Read the model definition and answer for the solid it produces. Units are mm, in the model's axes. A direction names the side the tool comes from. Give positions to 0.01 mm unless a question says otherwise; leave off trailing zeros. Order: outer loops, then holes, each group sorted by start corner. A loop starts at its lowest first (then second) coordinate and runs counter-clockwise, first axis right, second up. Notation, with made-up numbers: (72, -3.75) - (126, -3.75) arc R22 cw to (126, 10.25) - close; hole circle Ø10 at (70, 44.25). An arc over 180 degrees is marked (long way). Use a Markdown table: item, result. Add a question column.
1. For a pull along Y with two mould halves and no side action, classify faces 3 (the cylindrical face through (41, 3, 0)), 4 (the flat face through (29, 6, -15.218)), 5 (the flat face through (29, 8.5, -62)), 6 (the cylindrical face through (28.594, -0.003, -0.539)) as released by +Y, released by -Y, zero draft, split by the parting line, or undercut.
2. A cutting plane is placed at D-D on x = 25.5. Determine the outline of the cut face in (y, z).
3. A cutting plane is placed at C-C on y = -1.75. Determine the outline of the cut face in (x, z), and give its area (3 significant figures).
4. Which of the six approach directions +Z, -Z, +X, -X, +Y, -Y give full straight-line access (tool end or side, diameter ignored) to faces 1 (the cylindrical face through (28.59, -2.46, -27.39)), 2 (the flat face through (29, -13, -36))?
5. Flat-ended cylindrical pins translate along their axes: P1, Ø1.7, axis at x = 41, y = 5.5, coming from the -Z side; P2, Ø2.5, axis at x = 15, z = 0, coming from the +Y side; P3, Ø1, axis at x = 6, z = -7, coming from the -Y side; P4, Ø10, axis at x = 21, z = -8.5, coming from the -Y side. Find the tip coordinate at first contact, or state that the pin passes through.
6. Consider L1, parallel to X at y = 2.9, z = 0; L2, parallel to Y at x = 26.5, z = -69; L3, parallel to Z at x = 44, y = 11.5. Determine where each line is inside the solid, lowest interval first.
7. A cutting plane is placed at B-B on x = 43. Determine the outline of the cut face in (y, z), and give its area (3 significant figures).
8. A cutting plane is placed at A-A on z = 0. Determine the outline of the cut face in (x, y).
```python
from build123d import *

# Parameters (mm, degrees)
BOSS_EXTRUDE2_DEPTH     = 58
SKETCH4_R               = 2
CUT_EXTRUDE2_DEPTH      = 58
CUT_EXTRUDE2_DEPTH_BACK = 58


with BuildPart() as part:
    # Sketch3 → Boss-Extrude2 (new body)
    with BuildSketch(Plane(origin=(0, 0, 0), x_dir=(0, 0, -1), z_dir=(1, 0, 0))):
        with BuildLine():
            Line((-34.648232278, -14.351767722), (-38.183766184, -10.816233816))
            ThreePointArc((-38.183766184, -10.816233816), (-15.829835797, 2.627669894), (10.217922448, 4.024466625))
            Line((10.217922448, 4.024466625), (10.217922448, 13.5))
            Line((10.217922448, 13.5), (108, 13.5))
            Line((108, 13.5), (108, 8.5))
            Line((108, 8.5), (15.217922448, 8.5))
            Line((15.217922448, 8.5), (15.217922448, 2.811338878))
            ThreePointArc((15.217922448, 2.811338878), (27.556537728, -2.560391599), (38.183766184, -10.816233816))
            Line((38.183766184, -10.816233816), (34.648232278, -14.351767722))
            ThreePointArc((34.648232278, -14.351767722), (0, 0), (-34.648232278, -14.351767722))
        make_face()
    extrude(amount=BOSS_EXTRUDE2_DEPTH)

    # Sketch4 → Cut-Extrude2 (cut, two sides)
    with BuildSketch(Plane(origin=(0, 0, 0), x_dir=(1, 0, 0), z_dir=(0, 1, 0))) as cut_extrude2_sk:
        with Locations((15, 0)):
            Circle(SKETCH4_R)
        with Locations((43, 0)):
            Circle(SKETCH4_R)
    extrude(amount=CUT_EXTRUDE2_DEPTH, mode=Mode.SUBTRACT)
    extrude(cut_extrude2_sk.sketch, amount=-CUT_EXTRUDE2_DEPTH_BACK, mode=Mode.SUBTRACT)


solid = part.part
```
Output values:
| question | item | result |
|---|---|---|
| 1 | face 3 | zero draft |
| 1 | face 4 | undercut |
| 1 | face 5 | undercut |
| 1 | face 6 | released by -Y |
| 2 | outline | (-14.35, -34.65) - (-10.82, -38.18) arc R54 ccw to (2.81, -15.22) - (8.5, -15.22) - (8.5, -108) - (13.5, -108) - (13.5, -10.22) - (4.02, -10.22) arc R54 ccw to (-10.82, 38.18) - (-14.35, 34.65) arc R49 cw to start |
| 3 | outline | (0, -26.14) - (58, -26.14) - (58, -12.98) - (0, -12.98) - close; (0, 12.98) - (58, 12.98) - (58, 26.14) - (0, 26.14) - close |
| 3 | area | 1,530 mm² |
| 4 | face 1 | -Z, +X, -X |
| 4 | face 2 | -Z, +X, -X, -Y |
| 5 | P1 | z = -15.22 |
| 5 | P2 | through |
| 5 | P3 | y = -0.58 |
| 5 | P4 | y = -1.9 |
| 6 | L1 | 0 to 13, 17 to 41, 45 to 58 |
| 6 | L2 | 8.5 to 13.5 |
| 6 | L3 | -108 to -10.22 |
| 7 | outline | (-14.35, -34.65) - (-10.82, -38.18) arc R54 ccw to (2.81, -15.22) - (8.5, -15.22) - (8.5, -108) - (13.5, -108) - (13.5, -10.22) - (4.02, -10.22) arc R54 ccw to (4.96, -2) - (-0.04, -2) arc R49 cw to start; (-14.35, 34.65) arc R49 cw to (-0.04, 2) - (4.96, 2) arc R54 ccw to (-10.82, 38.18) - close |
| 7 | area | 899 mm² |
| 8 | outline | (0, 0) - (13, 0) - (13, 5) - (0, 5) - close; (17, 0) - (41, 0) - (41, 5) - (17, 5) - close; (45, 0) - (58, 0) - (58, 5) - (45, 5) - close |
